from build123d import *

# Parameters (mm, degrees)
SKETCH1_R                       = 5.5
BOSS_EXTRUDE1_DEPTH             = 67
SKETCH2_W                       = 1
SKETCH2_H                       = 1
CUT_EXTRUDE1_DEPTH              = 67
SKETCH3_R                       = 4.5
BOSS_EXTRUDE2_DEPTH             = 8
BOSS_EXTRUDE3_DEPTH             = 2
CHAMFER1_SIZE                   = 1
CHAMFER1_OF_MIRROR1_SIZE        = 1
F_3_0MM_DOWEL_HOLE1_D           = 3
F_3_0MM_DOWEL_HOLE1_CSINK_D     = 3.05
F_3_0MM_DOWEL_HOLE1_CSINK_ANGLE = 92


with BuildPart() as part:
    # Sketch1 → Boss-Extrude1 (new body)
    with BuildSketch(Plane.XY):
        Circle(SKETCH1_R)
    extrude(amount=BOSS_EXTRUDE1_DEPTH)

    # Sketch2 → Cut-Extrude1 (cut)
    with BuildSketch(Plane(origin=(0, 0, 0), x_dir=(-1, 0, 0), z_dir=(0, 0, -1))):
        with Locations((5.5, 0)):
            Rectangle(SKETCH2_W, SKETCH2_H)
        with Locations((-5.5, 0)):
            Rectangle(SKETCH2_W, SKETCH2_H)
    extrude(amount=-CUT_EXTRUDE1_DEPTH, mode=Mode.SUBTRACT)

    # Sketch3 → Boss-Extrude2 (add)
    with BuildSketch(Plane.XY.offset(67)):
        Circle(SKETCH3_R)
    boss_extrude2 = extrude(amount=BOSS_EXTRUDE2_DEPTH)

    # Sketch4 → Boss-Extrude3 (add)
    with BuildSketch(Plane.XY.offset(75)):
        with BuildLine():
            Line((-3.5, -0.992829401), (-3.5, 2.007170599))
            ThreePointArc((-3.5, 2.007170599), (0, 5.507170599), (3.5, 2.007170599))
            Line((3.5, 2.007170599), (3.5, -0.992829401))
            ThreePointArc((3.5, -0.992829401), (0, -4.492829401), (-3.5, -0.992829401))
        make_face()
    boss_extrude3 = extrude(amount=BOSS_EXTRUDE3_DEPTH)

    # Chamfer1
    chamfer1_edges = [part.edges().sort_by_distance(p)[0] for p in [
        (0, -4.492829401, 77),
        (3.5, 0.507170599, 77),
        (0, 5.507170599, 77),
        (-3.5, 0.507170599, 77),
    ]]
    chamfer(chamfer1_edges, length=CHAMFER1_SIZE)

    # Mirror1: Boss-Extrude2, Boss-Extrude3 across plane
    add(boss_extrude2.mirror(Plane.XY.offset(33.5)))
    add(boss_extrude3.mirror(Plane.XY.offset(33.5)))

    # Chamfer1 of Mirror1
    chamfer1_of_mirror1_edges = [part.edges().sort_by_distance(p)[0] for p in [
        (0, -4.492829401, -10),
        (3.5, 0.507170599, -10),
        (0, 5.507170599, -10),
        (-3.5, 0.507170599, -10),
    ]]
    chamfer(chamfer1_of_mirror1_edges, length=CHAMFER1_OF_MIRROR1_SIZE)

    # Ø3.0mm Dowel Hole1 (through all)
    with Locations(Plane(origin=(0, 0, -10), x_dir=(-1, 0, 0), z_dir=(0, 0, -1))):
        with Locations((0, 0)):
            CounterSinkHole(F_3_0MM_DOWEL_HOLE1_D / 2, F_3_0MM_DOWEL_HOLE1_CSINK_D / 2, counter_sink_angle=F_3_0MM_DOWEL_HOLE1_CSINK_ANGLE)


solid = part.part
The model under review builds one solid part; all positions refer to its coordinate system, in mm. A direction names the side the tool comes from. Round coordinates to 2 decimals unless told otherwise and drop trailing zeros. Write each loop counter-clockwise with the first axis right and the second up, starting at its lowest first coordinate (ties: lowest second). Pieces come first, ordered by that corner, then holes. Notation, with made-up numbers: M 24,68.25 L 44,68.25 A24 cw 44,107.25 Z; hole C -15,-11.75 d6. An arc over 180 degrees is marked long. Use a Markdown table: item, result. Add a question column.
Q1. The part is to be moulded in two halves that separate along Y. For faces 1 (the face through (-1.5, 0.07, 34.12)), 2 (the face through (-0.058, 4.666, 76.84)), 3 (the face through (0, 5, -8)), say which applies: pulls with the +Y half, pulls with the -Y half, needs draft (parallel to the pull), parting line crosses it, or undercut.
Q2. Insertion check: pin 1 (4 mm diameter, centred on x = -0.5, z = 56, fed in from -Y); pin 2 (6 mm diameter, centred on x = 1.5, z = 61, fed in from +Y); pin 3 (1.1 mm diameter, centred on y = 0.5, z = -8.5, fed in from +X); pin 4 (3 mm diameter, centred on x = 2.5, z = 22.5, fed in from +Y). Each pin has a flat end and moves straight along its axis. Give the tip position at first contact, or say it passes through.
Q3. To check wall thickness, follow line 1 (Y direction, x = 0, z = 59.5); line 2 (X direction, y = 0, z = 18.5); line 3 (Z direction, x = -2.5, y = -4.25). State the ranges of each line that lie inside material, in increasing order.
Q4. Machinability: for faces 4 (the face through (-0.077, 5.506, -8.493)), 5 (the face through (0.08, -4.49, -8.49)), 6 (the face through (0.08, -4.49, 75.49)), 7 (the face through (-0.59, 4.46, 70.94)), which of the approach directions +Z, -Z, +X, -X, +Y, -Y give a long, thin tool a straight path to every point of the face, cutting with its end or side? Answer none if there is none.
Q5. We need section C-C, the plane z = -3. State the section outline as (x, y) points.
Q6. We need section A-A, the plane z = 58.5. State the section outline as (x, y) points, plus the area to 3 significant figures.
Findings below:
| question | item | result |
|---|---|---|
| 1 | face 1 | undercut |
| 1 | face 2 | pulls with the +Y half |
| 1 | face 3 | needs draft |
| 2 | pin 1 | stops at y = -5.5 |
| 2 | pin 2 | stops at y = 5.5 |
| 2 | pin 3 | stops at x = 4.49 |
| 2 | pin 4 | stops at y = 5.41 |
| 3 | line 1 | y = -5.5 to -1.5, 1.5 to 5.5 |
| 3 | line 2 | x = -5 to -1.5, 1.5 to 5 |
| 3 | line 3 | z = 0 to 67 |
| 4 | face 4 | -Z, +Y |
| 4 | face 5 | -Z, -Y |
| 4 | face 6 | +Z, -Y |
| 4 | face 7 | none |
| 5 | outline | C 0,0 d9; hole C 0,0 d3 |
| 6 | outline | M -5.48,-0.5 A5.5 ccw 5.48,-0.5 L 5,-0.5 L 5,0.5 L 5.48,0.5 A5.5 ccw -5.48,0.5 L -5,0.5 L -5,-0.5 Z; hole C 0,0 d3 |
| 6 | area | 87.0 mm² |
